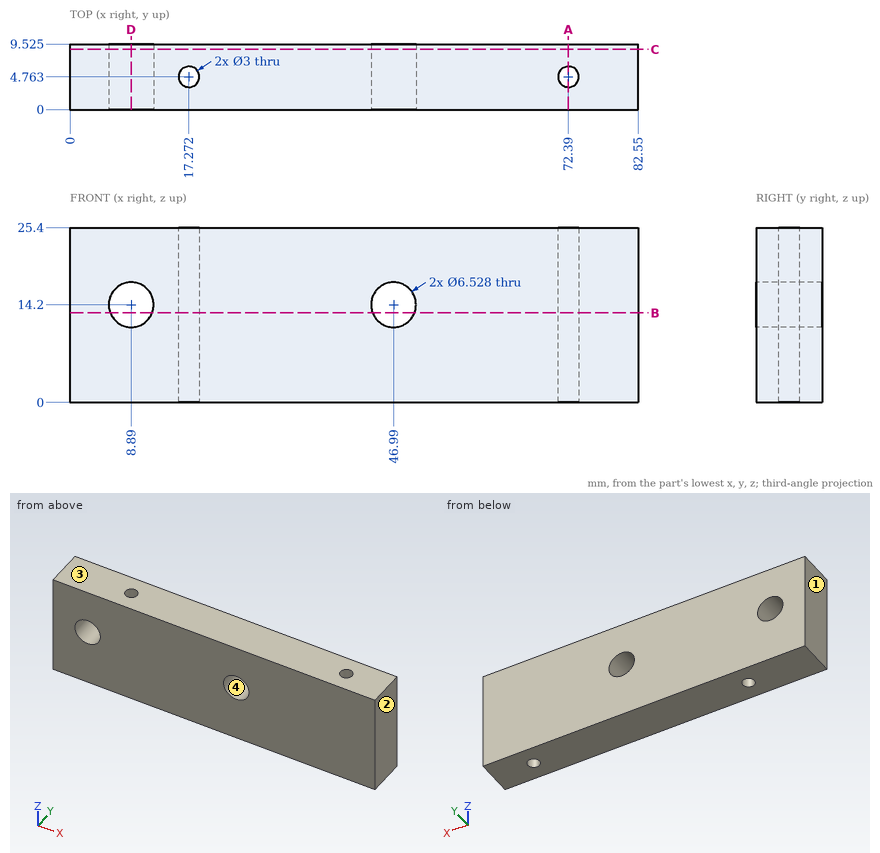
Input: dimensioned drawing with shaded views. Units: mm. Origin: part minimum x, y, z. Round coordinates to 2 decimals unless told otherwise and drop trailing zeros. Order: outer loops, then holes, each group sorted by start corner. A loop starts at its lowest first (then second) coordinate and runs counter-clockwise, first axis right, second up. Notation, with made-up numbers: M 27,62 L 68,62 A28 cw 68,80 Z; hole C -23,32 d5. An arc over 180 degrees is marked long. Use one line per item in the form item = value. Start each with the question number.
Q1. Cut plane D-D (x = 8.89). Return loops of the section in (y, z) (1 decimal), and give its area (3 significant figures).
Q2. Pin query (flat end, axial travel): pin 1 Ø3.5 at (x, y) = (72.39, 4.76) entering from -Z. Return the tip coordinate at first contact, or that it passes through.
Q3. Cut plane B-B (z = 13). Count the separate pieces of the cut face and the enclosed holes in it.
Q4. Mould query, pull axis X, two halves, no side actions, for the marked faces 1, 2, 3 and 4. Classes: +X half, -X half, draft (parallel to the pull), parting line (faces both ways), or undercut.
Q5. Material intervals for line 1 (Y direction, x = 72.39, z = 6.25) (1 decimal); line 2 (Z direction, x = 8.89, y = 3.25); line 3 (Z direction, x = 10.5, y = 1.25), sorted ascending. Write a range as [from, to].
Q6. Cut plane C-C (y = 8.75). Return loops of the section in (x, z), and give its area (3 significant figures).
Q7. Cut plane A-A (x = 72.39). Return loops of the section in (y, z) (1 decimal), and give its area (3 significant figures).
Geometry results:
q1.outline = M 0,0 L 9.5,0 L 9.5,10.9 L 0,10.9 Z; M 0,17.5 L 9.5,17.5 L 9.5,25.4 L 0,25.4 Z
q1.area = 180 mm^2
q2.pin_1 = 0
q3.separate_pieces = 3
q3.enclosed_holes = 2
q4.face_1 = -X half
q4.face_2 = +X half
q4.face_3 = draft
q4.face_4 = undercut
q5.line_1 = [0, 3.3], [6.3, 9.5]
q5.line_2 = [0, 10.94], [17.46, 25.4]
q5.line_3 = [0, 11.36], [17.04, 25.4]
q6.outline = M 0,0 L 82.55,0 L 82.55,25.4 L 0,25.4 Z; hole C 8.89,14.2 d6.53; hole C 46.99,14.2 d6.53
q6.area = 2,030 mm^2
q7.outline = M 0,0 L 3.3,0 L 3.3,25.4 L 0,25.4 Z; M 6.3,0 L 9.5,0 L 9.5,25.4 L 6.3,25.4 Z
q7.area = 166 mm^2
